Autodesk Inventor part; units mm, degrees
ref_plane "YZ Plane" through (0, 0, 0) normal (1, 0, 0) x (0, 1, 0)
ref_plane "XZ Plane" through (0, 0, 0) normal (0, 1, 0) x (-1, 0, 0)
ref_plane "XY Plane" through (0, 0, 0) normal (0, 0, 1) x (1, 0, 0)
sketch "Skizze3" plane through (0, 0, 0) normal (1, 0, 0) x (0, 1, 0)
  line L0 (0, 0) -> (4.4378, 0)
  line L1 (0, 1.5) -> (3, 1.5)
  line L2 (3, 1.5) -> (3, 2.5)
  line L3 (3, 2.5) -> (1, 2.5)
  line L4 (1, 2.5) -> (1, 4)
  line L5 (1, 4) -> (0, 4)
  line L6 (0, 4) -> (0, 1.5)
  dimension "d4" = 1
  dimension "d5" = 3
  dimension "d6" = 3
  dimension "d7" = 8
  dimension "d8" = 5
revolve "Umdrehung1" add sketch "Skizze3" angle 360 about axis through (0, 0, 0) along (0, 1, 0)
chamfer "Fase1" distance 0.2 angle 45 4 edges at (0, 3, -2.5) (0, 3, -1.5) (0, 1, -4) (0, 0, -1.5)
properties part number "BT014_huenin20_23" material "Messing"
CAD build for the part. Positions are in the model's coordinates, mm. A direction names the side the tool comes from. Give positions to 0.01 mm unless a question says otherwise; leave off trailing zeros. Loops run counter-clockwise (first coordinate to the right, second up) from the corner with the lowest first, then second, coordinate; pieces in that order, holes last. Notation, with made-up numbers: M -11,11 L 11,11 A24 cw 11,23 Z; hole C 33,-30.5 d1. An arc over 180 degrees is marked long. Use one line per item in the form item = value.
Item 1: Slice it at A-A (z = 0). List the corners of the cut face in (x, y), plus the area to 3 significant figures.
Determined:
outline = M -4,0 L -1.7,0 L -1.5,0.2 L -1.5,2.8 L -1.7,3 L -2.3,3 L -2.5,2.8 L -2.5,1 L -3.8,1 L -4,0.8 Z; M 1.5,0.2 L 1.7,0 L 4,0 L 4,0.8 L 3.8,1 L 2.5,1 L 2.5,2.8 L 2.3,3 L 1.7,3 L 1.5,2.8 Z
area = 8.84 mm2
Item 2: Drill centre lines: probe 1 along X at (y, z) = (1.7, 0); probe 2 along Y at (x, z) = (3, -1.5); probe 3 along Z at (x, y) = (0.5, 0.65). Where is each one in solid material? Low to high. Write a range as from..to.
Determined:
probe_1 = -2.5..-1.5, 1.5..2.5
probe_2 = 0..1
probe_3 = -3.97..-1.41, 1.41..3.97
Item 3: Flat gauge pins, fed straight in: pin 1 (4 mm diameter, centred on x = 0, z = 0, fed in from +Y); pin 2 (1.5 mm diameter, centred on x = -2.5, y = 1, fed in from -Z); pin 3 (1.5 mm diameter, centred on y = 2.5, z = 1.5, fed in from -X). Where does each tip first touch, or does it go through?
Determined:
pin_1 = 3
pin_2 = -3.58
pin_3 = -2.38
Item 4: Which spindle directions (+Z, -Z, +X, -X, +Y, -Y) get a long thin tool onto all of the face, cutting with end or side? Do faces 4 (the face through (3.905, 0.394, -0.867)), 5 (the face through (-2.5, 1, -0.9)). Say none if no direction does.
Determined:
face_4 = +Y, -Y
face_5 = +Y
Item 5: Slice it at B-B (y = 1.55). List the corners of the cut face in (x, z), plus the area to 3 significant figures.
Determined:
outline = C 0,0 d5; hole C 0,0 d3
area = 12.6 mm2
Item 6: Two-plate mould, pull along Z, no slides. Class faces 1 (the face through (0.07, 1.52, -1.5)), 2 (the face through (0, 0, 2)), 3 (the face through (2.44, 1.89, -0.54)): pulls with the +Z half, pulls with the -Z half, needs draft (parallel to the pull), parting line crosses it, or undercut.
Determined:
face_1 = undercut
face_2 = needs draft
face_3 = parting line crosses it
